```python
from build123d import *

# Parameters (mm, degrees)
F2_R      = 38.1
F3_DEPTH  = 147.6375
F4_R      = 0.127
F7_D      = 23.41626
F7_DEPTH  = 38.1
F7_START  = 1.0887055
F7_TIP    = 7.0349542395
F10_D     = 23.41626
F10_DEPTH = 38.1
F10_START = 1.0887055
F10_TIP   = 7.0349542395


with BuildPart() as f1:
    # F0 (on Right) → F1 (revolve)
    with BuildSketch(Plane.YZ):
        Polygon((0, 57.15), (0, 0), (147.6375, 0), (147.6375, 57.15), (144.5895, 57.15), (144.5895, 54.1528), (139.8397, 54.1528), (139.8397, 57.15), (136.8425, 57.15), (136.8425, 54.1528), (132.0927, 54.1528), (132.0927, 57.15), (127.3175, 57.15), (127.3175, 63.5), (20.32, 63.5), (20.32, 57.15), (15.5448, 57.15), (15.5448, 54.1528), (10.795, 54.1528), (10.795, 57.15), (7.7978, 57.15), (7.7978, 54.1528), (3.048, 54.1528), (3.048, 57.15), align=None)
    revolve(axis=Axis((0, 73.81875, 0), (0, 1, 0)))

    # F2 (on face) → F3 (cut, through all)
    with BuildSketch(Plane.XZ):
        Circle(F2_R)
    extrude(amount=-F3_DEPTH, mode=Mode.SUBTRACT)

    # F4
    f4_edges = [f1.edges().sort_by_distance(p)[0] for p in [
        (0, 0, -57.15),
        (0, 147.6375, -57.15),
    ]]
    fillet(f4_edges, radius=F4_R)

    # F7
    # its depths count from where the whole tool has entered the part; down to there all is cleared
    with Locations(Plane.YZ.offset(63.5).offset(-F7_START)):
        with Locations((73.81875, 0)):
            Hole(F7_D / 2, depth=F7_DEPTH)
            with Locations((0, 0, -(F7_DEPTH + F7_TIP / 2))):  # 118° drill point
                Cone(0, F7_D / 2, F7_TIP, mode=Mode.SUBTRACT)

    # F10
    # its depths count from where the whole tool has entered the part; down to there all is cleared
    with Locations(Plane(origin=(-63.5, 0, 0), x_dir=(0, 1, 0), z_dir=(-1, 0, 0)).offset(-F10_START)):
        with Locations((73.81875, 0)):
            Hole(F10_D / 2, depth=F10_DEPTH)
            with Locations((0, 0, -(F10_DEPTH + F10_TIP / 2))):  # 118° drill point
                Cone(0, F10_D / 2, F10_TIP, mode=Mode.SUBTRACT)


solid = f1.part
```
The model under review builds one solid part; all positions refer to its coordinate system, in mm. A direction names the side the tool comes from. Round coordinates to 2 decimals unless told otherwise and drop trailing zeros. Order: outer loops, then holes, each group sorted by start corner. A loop starts at its lowest first (then second) coordinate and runs counter-clockwise, first axis right, second up. Notation, with made-up numbers: M -31,81.25 L 2,81.25 A19 ccw 2,99.25 Z; hole C 7,32 d1. An arc over 180 degrees is marked long. Use a Markdown table: item, result.
1) Tool access review of faces 4 (the face through (-51, 144.59, 21)), 5 (the face through (2.513, 138.32, -57.095)), 6 (the face through (-49.688, 85.516, -0.515)): name each direction out of +Z, -Z, +X, -X, +Y, -Y from which nothing blocks a thin tool from reaching the whole face with its end or side.
Report:
| item | result |
|---|---|
| face 4 | none |
| face 5 | +Y |
| face 6 | +X, -X |
2) Insertion check: pin 1 (8 mm diameter, centred on y = 116, z = 45.5, fed in from +X); pin 2 (4 mm diameter, centred on y = 123, z = 27.5, fed in from +X); pin 3 (12 mm diameter, centred on x = -50.5, y = 101, fed in from -Z). Each pin has a flat end and moves straight along its axis. Give the tip position at first contact, or say it passes through.
Report:
| item | result |
|---|---|
| pin 1 | x = 48.06 |
| pin 2 | x = 58.15 |
| pin 3 | z = -45.3 |
3) Draft analysis for pull direction Y (two halves, no side actions). For faces 1 (the face through (2.513, 146.03, -57.095)), 2 (the face through (10, 20.32, -57)), 3 (the face through (-51, 139.84, -21)), state which applies: released by +Y, released by -Y, zero draft, split by the parting line, or undercut.
Report:
| item | result |
|---|---|
| face 1 | zero draft |
| face 2 | released by -Y |
| face 3 | undercut |
4) Consider section A-A (z = 0). Give the number of separate pieces and of enclosed holes in the cut face, then the cut area to 3 significant figures.
Report:
| item | result |
|---|---|
| separate pieces | 4 |
| enclosed holes | 0 |
| area | 5,680 mm^2 |
5) Consider section B-B (y = 107). Write out the cut boundary in (x, z).
Report:
| item | result |
|---|---|
| outline | C 0,0 d127; hole C 0,0 d76.2 |
6) Wall thickness on line 1 along Y through (x, z) = (13, -55) (1 decimal); line 2 along Y through (x, z) = (47.5, 0); line 3 along Y through (x, z) = (56.25, 0) (1 decimal): over which ranges is each line inside the solid? List them lowest first. Write a range as [from, to].
Report:
| item | result |
|---|---|
| line 1 | [0, 3], [7.8, 10.8], [15.5, 132.1], [136.8, 139.8], [144.6, 147.6] |
| line 2 | [0, 62.11], [85.53, 147.64] |
| line 3 | [0, 3], [7.8, 10.8], [15.5, 62.1], [85.5, 132.1], [136.8, 139.8], [144.6, 147.6] |
7) Consider section C-C (y = 13). Write out the cut boundary in (x, z), then the cut area to 3 significant figures.
Report:
| item | result |
|---|---|
| outline | C 0,0 d108.31; hole C 0,0 d76.2 |
| area | 4,650 mm^2 |
